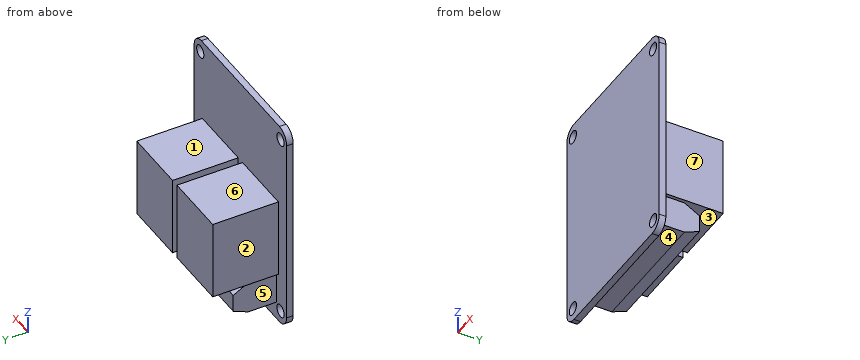
Autodesk Inventor part; units mm, degrees
ref_plane "YZ Plane" through (0, 0, 0) normal (1, 0, 0) x (0, 1, 0)
ref_plane "XZ Plane" through (0, 0, 0) normal (0, 1, 0) x (-1, 0, 0)
ref_plane "XY Plane" through (0, 0, 0) normal (0, 0, 1) x (1, 0, 0)
sketch "스케치2" plane through (0, 0, 0) normal (0, 1, 0) x (-1, 0, 0)
  line L0 (-16.35, -25.35) -> (16.35, -25.35)
  line L1 (19.35, -22.35) -> (19.35, 22.35)
  line L2 (16.35, 25.35) -> (-16.35, 25.35)
  line L3 (-19.35, 22.35) -> (-19.35, -22.35)
  line L4 (-19.35, -25.35) -> (19.35, 25.35) construction
  line L5 (19.35, -25.35) -> (-19.35, 25.35) construction
  circle A0 centre (16.8, 22.25) radius 1.5
  line L6 (0, 0) -> (0, -6.2498)
  line L7 (0, 0) -> (4.685, 0)
  circle A1 centre (16.8, -22.25) radius 1.5
  circle A2 centre (-16.8, 22.25) radius 1.5
  circle A3 centre (-16.8, -22.25) radius 1.5
  arc A4 (19.35, 22.35) -> (16.35, 25.35) centre (16.35, 22.35) ccw
  arc A5 (16.35, -25.35) -> (19.35, -22.35) centre (16.35, -22.35) ccw
  arc A6 (-19.35, -22.35) -> (-16.35, -25.35) centre (-16.35, -22.35) ccw
  arc A7 (-16.35, 25.35) -> (-19.35, 22.35) centre (-16.35, 22.35) ccw
  dimension "d0" = 38.7
  dimension "d1" = 50.7
  dimension "d2" = 3
  dimension "d4" = 44.5
  dimension "d5" = 3
  dimension "d24" = 33.6
extrude "돌출1" add sketch "스케치2" along normal blind 1.55
sketch "스케치3" plane through (0, 1.55, 0) normal (0, 1, 0) x (1, 0, 0)
  line L0 (-15.9, -5.45) -> (-0.9, -5.45)
  line L1 (-0.9, -5.45) -> (-0.9, 13.35)
  line L2 (-0.9, 13.35) -> (-15.9, 13.35)
  line L3 (-15.9, 13.35) -> (-15.9, -5.45)
  line L4 (-15.9, -5.45) -> (-0.9, 13.35) construction
  line L5 (-0.9, -5.45) -> (-15.9, 13.35) construction
  line L6 (16.35, 25.35) -> (-16.35, 25.35)
  line L7 (0, 0) -> (0, -13.7943)
  line L8 (15.9, -5.45) -> (0.9, -5.45)
  line L9 (0.9, -5.45) -> (0.9, 13.35)
  line L10 (0.9, 13.35) -> (15.9, 13.35)
  line L11 (15.9, 13.35) -> (15.9, -5.45)
  line L12 (15.9, -5.45) -> (0.9, 13.35) construction
  line L13 (0.9, -5.45) -> (15.9, 13.35) construction
  point P0 (-8.4, 3.95)
  point P1 (8.4, 3.95)
  dimension "d8" = 15
  dimension "d9" = 18.8
  dimension "d10" = 0.9
  dimension "d11" = 12
extrude "돌출2" add sketch "스케치3" along normal blind 15.4
sketch "스케치4" plane through (0, 0, 0) normal (1, 0, 0) x (0, 1, 0)
  line L0 (1.55, -22.35) -> (1.55, 22.35)
  line L1 (11.75, -13.45) -> (1.55, -13.45)
  line L2 (1.55, -13.45) -> (1.55, -21.05)
  line L3 (1.55, -21.05) -> (11.75, -21.05)
  line L4 (11.75, -21.05) -> (11.75, -13.45)
  line L5 (0, -25.35) -> (1.55, -25.35)
  line L6 (11.75, -19.55) -> (8.25, -21.05)
  line L7 (1.55, -13.35) -> (16.95, -13.35)
  line L8 (8.25, -13.45) -> (11.75, -15.45)
  point P0 (0, 0)
  point P1 (1.55, -13.45)
  dimension "d16" = 7.6
  dimension "d17" = 10.2
  dimension "d18" = 4.3
  dimension "d19" = 1.5
  dimension "d20" = 2
  dimension "d21" = 3.5
extrude "돌출3" add sketch "스케치4" along normal mid plane 30.4 contours L0 L1 L8 L4 L6 L3
properties part number "더블 릴레이 모듈"
Check sheet for the modelled part. Datum: model origin and axes. Units: mm. Face numbers are marked on the shaded views. A direction names the side the tool comes from. Coordinates: 2 decimals unless noted, no trailing zeros. Write each loop counter-clockwise with the first axis right and the second up, starting at its lowest first coordinate (ties: lowest second). Pieces come first, ordered by that corner, then holes. Notation, with made-up numbers: (68.25, 30) -> (112.25, 30) arc R21 cw to (112.25, 53) -> close; hole circle Ø2 at (47, 14.25). An arc over 180 degrees is marked (long way). Use a Markdown table: item, result.
1. Sectioned sample at A-A (y = 6.75). Enter the section's corners in (x, z).
Reported:
| item | result |
|---|---|
| outline | (-15.9, -13.35) -> (-0.9, -13.35) -> (-0.9, 5.45) -> (-15.9, 5.45) -> close; (-15.2, -21.05) -> (15.2, -21.05) -> (15.2, -13.45) -> (-15.2, -13.45) -> close; (0.9, -13.35) -> (15.9, -13.35) -> (15.9, 5.45) -> (0.9, 5.45) -> close |
2. Tool access check on the marked faces 5, 6 and 7. Record the directions out of +Z, -Z, +X, -X, +Y, -Y that give a thin tool (end or side, any length) a straight path to the whole face; none if there is none.
Reported:
| item | result |
|---|---|
| face 5 | -Z, -X, +Y |
| face 6 | +Z, +X, -X, +Y |
| face 7 | +Z, -Z, +X, +Y |
3. Release check for a two-part mould opening along Z. For the marked faces 1, 2, 3 and 4 record: pulls with the +Z half, pulls with the -Z half, needs draft (parallel to the pull), parting line crosses it, or undercut.
Reported:
| item | result |
|---|---|
| face 1 | pulls with the +Z half |
| face 2 | needs draft |
| face 3 | undercut |
| face 4 | pulls with the -Z half |
4. Go/stop test with flat-tipped pins: pin 1 Ø4 at (x, y) = (-3.5, 11) entering from +Z; pin 2 Ø4 at (y, z) = (8, -18) entering from -X; pin 3 Ø2 at (x, z) = (-7.5, -17) entering from +Y. Record where each tip stops, or that it passes through.
Reported:
| item | result |
|---|---|
| pin 1 | stops at z = 5.45 |
| pin 2 | stops at x = -15.2 |
| pin 3 | stops at y = 11.75 |
5. Sectioned sample at B-B (x = 11.5). Enter the section's corners in (y, z), plus the area to 4 significant figures.
Reported:
| item | result |
|---|---|
| outline | (0, -25.35) -> (1.55, -25.35) -> (1.55, -21.05) -> (8.25, -21.05) -> (11.75, -19.55) -> (11.75, -15.45) -> (8.25, -13.45) -> (1.55, -13.45) -> (1.55, -13.35) -> (16.95, -13.35) -> (16.95, 5.45) -> (1.55, 5.45) -> (1.55, 25.35) -> (0, 25.35) -> close |
| area | 439.5 mm2 |
6. Sectioned sample at D-D (y = 11). Enter the section's corners in (x, z), plus the area to 3 significant figures.
Reported:
| item | result |
|---|---|
| outline | (-15.9, -13.35) -> (-0.9, -13.35) -> (-0.9, 5.45) -> (-15.9, 5.45) -> close; (-15.2, -19.87) -> (15.2, -19.87) -> (15.2, -15.02) -> (-15.2, -15.02) -> close; (0.9, -13.35) -> (15.9, -13.35) -> (15.9, 5.45) -> (0.9, 5.45) -> close |
| area | 711 mm2 |
7. Scan lines: line 1 along X through (y, z) = (6.5, -5.5); line 2 along Z through (x, y) = (-16.8, 0.65); line 3 along Y through (x, z) = (-4, 17). Record each from-to range of solid material in increasing order.
Reported:
| item | result |
|---|---|
| line 1 | x = -15.9 to -0.9, 0.9 to 15.9 |
| line 2 | z = -25.32 to -23.75, -20.75 to 20.75, 23.75 to 25.32 |
| line 3 | y = 0 to 1.55 |
8. Sectioned sample at C-C (z = 4.5). Enter the section's corners in (x, y), plus the area to 3 significant figures.
Reported:
| item | result |
|---|---|
| outline | (-19.35, 0) -> (19.35, 0) -> (19.35, 1.55) -> (15.9, 1.55) -> (15.9, 16.95) -> (0.9, 16.95) -> (0.9, 1.55) -> (-0.9, 1.55) -> (-0.9, 16.95) -> (-15.9, 16.95) -> (-15.9, 1.55) -> (-19.35, 1.55) -> close |
| area | 522 mm2 |
